The model under review builds one solid part; all positions refer to its coordinate system, in mm. A direction names the side the tool comes from. Round coordinates to 2 decimals unless told otherwise and drop trailing zeros. Loops run counter-clockwise (first coordinate to the right, second up) from the corner with the lowest first, then second, coordinate; pieces in that order, holes last. Notation, with made-up numbers: M -26.5,64.5 L 15.5,64.5 A36 ccw 15.5,99.5 Z; hole C 66,9 d10. An arc over 180 degrees is marked long. One line per question, with ' | ' between items.
from build123d import *

# Parameters (mm, degrees)
SKETCH_R           = 22.5
PAD_DEPTH          = 50
SKETCH002_R        = 2
PAD001_DEPTH       = 12
POLARPATTERN_COUNT = 3
CHAMFER_SIZE       = 3
FILLET_R           = 5
SKETCH001_R        = 17.9
POCKET_DEPTH       = 45
CHAMFER001_SIZE    = 1
CHAMFER002_SIZE    = 1
SKETCH003_R        = 2
POCKET001_DEPTH    = 22.501
CHAMFER003_SIZE    = 3


with BuildPart() as part:
    # Sketch (on XY_Plane of Origin) → Pad (new body)
    with BuildSketch(Plane.XY):
        Circle(SKETCH_R)
    extrude(amount=PAD_DEPTH)

    # Sketch002 (on Face2 of Pad) → Pad001 (join)
    with BuildSketch(Plane(origin=(0, 0, 0), x_dir=(1, 0, 0), z_dir=(0, 0, -1))):
        with BuildLine():
            ThreePointArc((0, 8), (-8, 0), (0, -8))
            Line((0, -8), (28, -8))
            ThreePointArc((28, -8), (36, 0), (28, 8))
            Line((0, 8), (28, 8))
        make_face()
        with Locations((28, 0)):
            Circle(SKETCH002_R, mode=Mode.SUBTRACT)
    pad001 = extrude(amount=-PAD001_DEPTH)

    # PolarPattern: Pad001 ×3 about axis
    polarpattern_axis = Axis((0, 0, 0), (0, 0, -1))
    for i in range(1, POLARPATTERN_COUNT):
        add(pad001.rotate(polarpattern_axis, i * 360 / POLARPATTERN_COUNT))

    # Chamfer
    chamfer_edges = [part.edges().sort_by_distance(p)[0] for p in [
        (26, 0, 12),
        (-13, 22.51666, 12),
        (-13, -22.51666, 12),
    ]]
    chamfer(chamfer_edges, length=CHAMFER_SIZE)

    # Fillet
    fillet_edges = [part.edges().sort_by_distance(p)[0] for p in [
        (21.029741, 8, 6),
        (-3.586667, 22.21229, 6),
        (-17.443074, 14.21229, 6),
        (-17.443074, -14.21229, 6),
        (-3.586667, -22.21229, 6),
        (21.029741, -8, 6),
    ]]
    fillet(fillet_edges, radius=FILLET_R)

    # Sketch001 (on Face3 of Pad) → Pocket (cut)
    with BuildSketch(Plane.XY.offset(50)):
        Circle(SKETCH001_R)
    extrude(amount=-POCKET_DEPTH, mode=Mode.SUBTRACT)

    # Chamfer001
    chamfer001_edges = [part.edges().sort_by_distance(p)[0] for p in [
        (-22.5, 0, 50),
        (-17.9, 0, 50),
    ]]
    chamfer(chamfer001_edges, length=CHAMFER001_SIZE)

    # Chamfer002
    chamfer002_edges = [part.edges().sort_by_distance(p)[0] for p in [
        (11.25, 19.485572, 0),
        (21.665965, 8.709418, 0),
        (-3.290405, 23.117985, 0),
        (26.116621, 8, 0),
        (-6.130107, 26.617657, 0),
        (36, 0, 0),
        (-18, 31.176915, 0),
        (26.116621, -8, 0),
        (-19.986514, 18.617657, 0),
        (21.665965, -8.709418, 0),
        (-18.37556, 14.408567, 0),
        (11.25, -19.485572, 0),
        (-22.5, 0, 0),
        (-3.290405, -23.117985, 0),
        (-18.37556, -14.408567, 0),
        (-6.130107, -26.617657, 0),
        (-19.986514, -18.617657, 0),
        (-18, -31.176915, 0),
        (-13, 22.51666, 0),
        (-13, -22.51666, 0),
        (26, 0, 0),
    ]]
    chamfer(chamfer002_edges, length=CHAMFER002_SIZE)

    # Sketch003 → Pocket001 (cut, through all)
    with BuildSketch(Plane.YZ):
        with Locations((0, 20)):
            Circle(SKETCH003_R)
        with Locations((0, 40)):
            Circle(SKETCH003_R)
    extrude(amount=-POCKET001_DEPTH, mode=Mode.SUBTRACT)

    # Chamfer003
    chamfer003_edges = [part.edges().sort_by_distance(p)[0] for p in [
        (-22.410935, -2, 40),
        (-22.410935, -2, 20),
    ]]
    chamfer(chamfer003_edges, length=CHAMFER003_SIZE)


solid = part.part
1) Insertion check: P1, Ø5, axis at y = 0, z = 40, coming from the -X side; P2, Ø16.5, axis at x = -9, y = -22.5, coming from the +Z side; P3, Ø6.5, axis at y = 0, z = 20, coming from the +X side; P4, Ø3, axis at x = -14, y = -24.25, coming from the +Z side. Each pin has a flat end and moves straight along its axis. Give the tip position at first contact, or say it passes through.
Output values:
P1: stops at x = -20 | P2: stops at z = 50 | P3: stops at x = 22.5 | P4: passes through
2) Add section B-B on x = -14. State how many separate pieces and enclosed holes the cut face has, then the cut area to 3 significant figures.
Output values:
separate pieces: 3 | enclosed holes: 0 | area: 989 mm²
3) Machinability: for faces 4 (the conical face through (35.2, -0.2, 0.2)), 5 (the flat face through (-19.97, -18.59, 6.42)), 6 (the cylindrical face through (-19, 0, 22)), which of the approach directions +Z, -Z, +X, -X, +Y, -Y give a long, thin tool a straight path to every point of the face, cutting with its end or side? Answer none if there is none.
Output values:
face 4: -Z, +X | face 5: +Z, -Z, -X | face 6: -X
4) For line 1 (X direction, y = 0, z = 35); line 2 (Z direction, x = 2.5, y = 4); line 3 (Y direction, x = 15, z = 21), list the stretches that pass through material, from the lowest coordinate up.
Output values:
line 1: x = -22.5 to -17.9, 17.9 to 22.5 | line 2: z = 0 to 5 | line 3: y = -16.77 to -9.77, 9.77 to 16.77
5) Mouldability with a two-part tool opening along X and no side actions: class faces 1 (the flat face through (1.5, -19, 50)), 2 (the cylindrical face through (20.784, -8.618, 29.997)), 3 (the cylindrical face through (29.908, -0.601, 4.944)) as +X half, -X half, draft (parallel to the pull), parting line (faces both ways), or undercut.
Output values:
face 1: draft | face 2: parting line | face 3: undercut
6) Add section A-A on z = 32. State the section outline as (x, y) points.
Output values:
outline: C 0,0 d45; hole C 0,0 d35.8
